Verification items for the finished model (mm, model axes). A direction names the side the tool comes from. Round coordinates to 2 decimals unless told otherwise and drop trailing zeros. Order: outer loops, then holes, each group sorted by start corner. A loop starts at its lowest first (then second) coordinate and runs counter-clockwise, first axis right, second up.
```python
from build123d import *

# Parameters (mm, degrees)
SKETCH1_R           = 2.5
BOSS_EXTRUDE1_DEPTH = 25
FILLET1_R           = 5


with BuildPart() as part:
    # Sketch1 → Boss-Extrude1 (new body)
    with BuildSketch(Plane.XY):
        with BuildLine():
            Line((-25, 10.583953595), (-25, -30))
            Line((-25, -30), (-10, -45))
            Line((-10, -45), (12.687018602, -45))
            Line((12.687018602, -45), (12.687018602, -43))
            Line((12.687018602, -43), (1, -43))
            Line((1, -43), (1, -4.387482194))
            ThreePointArc((1, -4.387482194), (3.181980515, 3.181980515), (-4.387482194, 1))
            Line((-4.387482194, 1), (-23, 1))
            Line((-23, 1), (-23, 10.583953595))
            Line((-23, 10.583953595), (-25, 10.583953595))
        make_face()
        Circle(SKETCH1_R, mode=Mode.SUBTRACT)
        with BuildLine():
            Line((-23, -29.171572875), (-9.171572875, -43))
            Line((-9.171572875, -43), (-1, -43))
            Line((-1, -43), (-1, -4.387482194))
            ThreePointArc((-1, -4.387482194), (-3.181980515, -3.181980515), (-4.387482194, -1))
            Line((-4.387482194, -1), (-23, -1))
            Line((-23, -1), (-23, -29.171572875))
        make_face(mode=Mode.SUBTRACT)
    extrude(amount=BOSS_EXTRUDE1_DEPTH)

    # Fillet1
    fillet1_edges = [part.edges().sort_by_distance(p)[0] for p in [
        (-10, -45, 12.5),
        (-25, -30, 12.5),
        (-23, -29.171572875, 12.5),
        (-9.171572875, -43, 12.5),
    ]]
    fillet(fillet1_edges, radius=FILLET1_R)


solid = part.part
```
1) Go/stop test with flat-tipped pins: pin 1 Ø5 at (x, z) = (-14.5, 4) entering from -Y; pin 2 Ø3 at (x, y) = (0, 0) entering from -Z; pin 3 Ø6.5 at (x, z) = (-3.5, 9) entering from +Y; pin 4 Ø1.5 at (y, z) = (-37.5, 8) entering from +X. Record where each tip stops, or that it passes through.
2) Sectioned sample at B-B on x = -5.5. Record the cut outline in (y, z).
3) Sectioned sample at D-D on x = 8. Record the cut outline in (y, z), then the cut area to 3 significant figures.
4) Sectioned sample at C-C on z = 7.5. Record the cut outline in (x, y), then the cut area to 3 significant figures.
5) Sectioned sample at A-A on y = -21. Record the cut outline in (x, z).
6) Tool access check on faces 4 (the cylindrical face through (-9.87, -44.61, 12.68)), 5 (the cylindrical face through (-9.04, -42.61, 12.68)), 6 (the flat face through (2, -45, 12)), 7 (the flat face through (1, -24, 12)), 8 (the flat face through (-23, 6, 12)). Record the directions out of +Z, -Z, +X, -X, +Y, -Y that give a thin tool (end or side, any length) a straight path to the whole face; none if there is none.
7) Scan lines: probe 1 along Y at (x, z) = (0, 8.25); probe 2 along Y at (x, z) = (-4.5, 6.75); probe 3 along X at (y, z) = (-21, 19.25). Record each from-to range of solid material in increasing order.
8) Draft check along X on faces 1 (the flat face through (-14, 1, 12)), 2 (the cylindrical face through (-24.63, -29.82, 12.68)), 3 (the flat face through (-0.7, -17.1, 0)). Enter one of: released by +X, released by -X, zero draft, split by the parting line, or undercut.
Returned:
1. pin 1: stops at y = -43
1. pin 2: passes through
1. pin 3: stops at y = 4.49
1. pin 4: stops at x = 1
2. outline: (-45, 0) - (-43, 0) - (-43, 25) - (-45, 25) - close; (-1, 0) - (1, 0) - (1, 25) - (-1, 25) - close
3. outline: (-45, 0) - (-43, 0) - (-43, 25) - (-45, 25) - close
3. area: 50.0 mm2
4. outline: (-25, -27.93) arc R5 ccw to (-23.54, -31.46) - (-11.46, -43.54) arc R5 ccw to (-7.93, -45) - (12.69, -45) - (12.69, -43) - (1, -43) - (1, -4.39) arc R4.5 ccw (long way) to (-4.39, 1) - (-23, 1) - (-23, 10.58) - (-25, 10.58) - close; hole (-23, -27.1) arc R5 ccw to (-21.54, -30.64) - (-10.64, -41.54) arc R5 ccw to (-7.1, -43) - (-1, -43) - (-1, -4.39) arc R4.5 cw to (-4.39, -1) - (-23, -1) - close; hole circle Ø5 at (0, 0)
4. area: 324 mm2
5. outline: (-25, 0) - (-23, 0) - (-23, 25) - (-25, 25) - close; (-1, 0) - (1, 0) - (1, 25) - (-1, 25) - close
6. face 4: +Z, -Z, -X, -Y
6. face 5: +Z, -Z
6. face 6: +Z, -Z, +X, -X, -Y
6. face 7: +Z, -Z, +X
6. face 8: +Z, -Z, +Y
7. probe 1: y = -45 to -2.5, 2.5 to 4.5
7. probe 2: y = -45 to -43, -1 to 1
7. probe 3: x = -25 to -23, -1 to 1
8. face 1: undercut
8. face 2: released by -X
8. face 3: zero draft
